from build123d import *

# Parameters (mm, degrees)
SKETCH2_R               = 1.75
BOSS_EXTRUDE1_DEPTH     = 10
SKETCH3_R               = 11.25
CUT_EXTRUDE1_DEPTH      = 9
SKETCH4_W               = 10
SKETCH4_H               = 5
CUT_EXTRUDE2_DEPTH      = 15
CUT_EXTRUDE2_DEPTH_BACK = 15
FILLET1_R               = 10


with BuildPart() as part:
    # Sketch2 → Boss-Extrude1 (new body)
    with BuildSketch(Plane(origin=(0, 0, 0), x_dir=(1, 0, 0), z_dir=(0, 1, 0))):
        with BuildLine():
            Line((-22.25, 4.465142775), (-6.3, 12.50239977))
            ThreePointArc((-6.3, 12.50239977), (0, 14), (6.3, 12.50239977))
            Line((6.3, 12.50239977), (22.25, 4.465142775))
            ThreePointArc((22.25, 4.465142775), (25, 0), (22.25, -4.465142775))
            Line((22.25, -4.465142775), (6.3, -12.50239977))
            ThreePointArc((6.3, -12.50239977), (0, -14), (-6.3, -12.50239977))
            Line((-6.3, -12.50239977), (-22.25, -4.465142775))
            ThreePointArc((-22.25, -4.465142775), (-25, 0), (-22.25, 4.465142775))
        make_face()
        with Locations((-20, 0)):
            Circle(SKETCH2_R, mode=Mode.SUBTRACT)
        with Locations((20, 0)):
            Circle(SKETCH2_R, mode=Mode.SUBTRACT)
    extrude(amount=BOSS_EXTRUDE1_DEPTH)

    # Sketch3 → Cut-Extrude1 (cut)
    with BuildSketch(Plane(origin=(0, 10, 0), x_dir=(1, 0, 0), z_dir=(0, 1, 0))):
        Circle(SKETCH3_R)
    extrude(amount=-CUT_EXTRUDE1_DEPTH, mode=Mode.SUBTRACT)

    # Sketch4 → Cut-Extrude2 (cut, two sides)
    with BuildSketch(Plane.XY) as cut_extrude2_sk:
        with Locations((-20, 7.5)):
            Rectangle(SKETCH4_W, SKETCH4_H)
        with Locations((20, 7.5)):
            Rectangle(SKETCH4_W, SKETCH4_H)
    extrude(amount=CUT_EXTRUDE2_DEPTH, mode=Mode.SUBTRACT)
    extrude(cut_extrude2_sk.sketch, amount=-CUT_EXTRUDE2_DEPTH_BACK, mode=Mode.SUBTRACT)

    # Fillet1
    fillet1_edges = [part.edges().sort_by_distance(p)[0] for p in [
        (-15, 7.5, -8.118441409),
        (15, 7.5, -8.118441409),
        (-15, 7.5, 8.118441409),
        (15, 7.5, 8.118441409),
    ]]
    fillet(fillet1_edges, radius=FILLET1_R)


solid = part.part
Check sheet for the modelled part. Datum: model origin and axes. Units: mm. A direction names the side the tool comes from. Give positions to 0.01 mm unless a question says otherwise; leave off trailing zeros. Loops run counter-clockwise (first coordinate to the right, second up) from the corner with the lowest first, then second, coordinate; pieces in that order, holes last. Notation, with made-up numbers: M 63,-32 L 95,-32 A15 cw 95,-25 Z; hole C 16.5,70 d2. An arc over 180 degrees is marked long. Use a Markdown table: item, result. Add a question column.
Q1. Tool access check on faces 1 (the cylindrical face through (-13.474, 7.465, 7.269)), 2 (the cylindrical face through (5.19, 5.56, 9.98)), 3 (the cylindrical face through (13.474, 7.465, -7.269)). Record the directions out of +Z, -Z, +X, -X, +Y, -Y that give a thin tool (end or side, any length) a straight path to the whole face; none if there is none.
Q2. Sectioned sample at C-C, the plane y = 4. Record the cut outline in (x, z), then the cut area to 3 significant figures.
Q3. Go/stop test with flat-tipped pins: pin 1 (5.5 mm diameter, centred on x = -20, z = 0, fed in from +Y); pin 2 (3 mm diameter, centred on x = -4, y = 5, fed in from -Z) (3 decimals); pin 3 (13.5 mm diameter, centred on x = 0, z = 0, fed in from +Y). Record where each tip stops, or that it passes through.
Q4. Sectioned sample at D-D, the plane x = 0. Record the cut outline in (y, z).
Q5. Mould release check, pull along Z, two halves, no side actions. Record for faces 4 (the cylindrical face through (-21.75, 2.46, -0.08)), 5 (the cylindrical face through (13.474, 7.465, 7.269)), 6 (the cylindrical face through (25, 2, 0)), 7 (the flat face through (12.391, 3.819, -9.433)): pulls with the +Z half, pulls with the -Z half, needs draft (parallel to the pull), parting line crosses it, or undercut.
Q6. Sectioned sample at A-A, the plane y = 0.5. Record the cut outline in (x, z), then the cut area to 3 significant figures.
Q7. Scan lines: line 1 along X through (y, z) = (3.55, 0); line 2 along X through (y, z) = (9, -0.25); line 3 along X through (y, z) = (2, 0.75). Record each from-to range of solid material in increasing order. Write a range as [from, to].
Q8. Sectioned sample at B-B, the plane z = 0. Record the cut outline in (x, y), then the cut area to 4 significant figures.
Verdict:
| question | item | result |
|---|---|---|
| 1 | face 1 | +Z, -X, +Y |
| 1 | face 2 | +Y |
| 1 | face 3 | -Z, +X, +Y |
| 2 | outline | M -22.25,-4.47 L -6.3,-12.5 A14 ccw 6.3,-12.5 L 22.25,-4.47 A5 ccw 22.25,4.47 L 6.3,12.5 A14 ccw -6.3,12.5 L -22.25,4.47 A5 ccw Z; hole C -20,0 d3.5; hole C 0,0 d22.5; hole C 20,0 d3.5 |
| 2 | area | 500 mm^2 |
| 3 | pin 1 | y = 5 |
| 3 | pin 2 | z = -13.775 |
| 3 | pin 3 | y = 1 |
| 4 | outline | M 0,-14 L 10,-14 L 10,-11.25 L 1,-11.25 L 1,11.25 L 10,11.25 L 10,14 L 0,14 Z |
| 5 | face 4 | undercut |
| 5 | face 5 | pulls with the +Z half |
| 5 | face 6 | parting line crosses it |
| 5 | face 7 | pulls with the -Z half |
| 6 | outline | M -22.25,-4.47 L -6.3,-12.5 A14 ccw 6.3,-12.5 L 22.25,-4.47 A5 ccw 22.25,4.47 L 6.3,12.5 A14 ccw -6.3,12.5 L -22.25,4.47 A5 ccw Z; hole C -20,0 d3.5; hole C 20,0 d3.5 |
| 6 | area | 898 mm^2 |
| 7 | line 1 | [-25, -21.75], [-18.25, -11.25], [11.25, 18.25], [21.75, 25] |
| 7 | line 2 | [-15, -11.25], [11.25, 15] |
| 7 | line 3 | [-24.94, -21.58], [-18.42, -11.22], [11.22, 18.42], [21.58, 24.94] |
| 8 | outline | M -25,0 L -21.75,0 L -21.75,5 L -25,5 Z; M -18.25,0 L 18.25,0 L 18.25,5 L 15,5 L 15,10 L 11.25,10 L 11.25,1 L -11.25,1 L -11.25,10 L -15,10 L -15,5 L -18.25,5 Z; M 21.75,0 L 25,0 L 25,5 L 21.75,5 Z |
| 8 | area | 162.5 mm^2 |
